from build123d import *

# Parameters (mm, degrees)
SKETCH1_R           = 2.286
BOSS_EXTRUDE1_DEPTH = 6.35
CHAMFER1_SIZE       = 17.78
CHAMFER1_SIZE2      = 26.652616032
FILLET1_R           = 3.81


with BuildPart() as part:
    # Sketch1 → Boss-Extrude1 (new body)
    with BuildSketch(Plane.XY):
        Polygon((-34.167492812, 55.206788795), (-6.35, 37.482986116), (-6.35, -6.35), (6.35, -6.35), (6.35, 44.45), (-27.343211205, 65.917492812), align=None)
        Circle(SKETCH1_R, mode=Mode.SUBTRACT)
        with Locations((0, 38.1)):
            Circle(SKETCH1_R, mode=Mode.SUBTRACT)
        with Locations((-25.4, 57.15)):
            Circle(SKETCH1_R, mode=Mode.SUBTRACT)
    extrude(amount=BOSS_EXTRUDE1_DEPTH)

    # Chamfer1
    chamfer1_edges = [part.edges().sort_by_distance(p)[0] for p in [
        (-6.35, 37.482986116, 3.175),
    ]]
    chamfer1_side = [part.faces().sort_by_distance(p)[0] for p in [
        (-20.258746406, 46.344887456, 3.175),
    ]]
    chamfer(chamfer1_edges, length=CHAMFER1_SIZE, length2=CHAMFER1_SIZE2, reference=chamfer1_side[0])

    # Fillet1
    fillet1_edges = [part.edges().sort_by_distance(p)[0] for p in [
        (-27.343211205, 65.917492812, 3.175),
        (6.35, 44.45, 3.175),
        (6.35, -6.35, 3.175),
        (-6.35, -6.35, 3.175),
        (-34.167492812, 55.206788795, 3.175),
        (-6.35, 10.830370085, 3.175),
        (-21.344985624, 47.036980366, 3.175),
    ]]
    fillet(fillet1_edges, radius=FILLET1_R)


solid = part.part
Check sheet for the modelled part. Datum: model origin and axes. Units: mm. A direction names the side the tool comes from. Give positions to 0.01 mm unless a question says otherwise; leave off trailing zeros. Loops run counter-clockwise (first coordinate to the right, second up) from the corner with the lowest first, then second, coordinate; pieces in that order, holes last. Notation, with made-up numbers: M -25,21 L 7,21 A26 cw 7,35 Z; hole C 69,-0.75 d9. An arc over 180 degrees is marked long. Answer as a JSON object with one key per item and string values. Group by question number.
Q1. Cross-section at A-A on y = 0. Record the cut outline in (x, z).
Q2. Go/stop test with flat-tipped pins: P1, Ø5.5, axis at x = 0, y = 38.1, coming from the -Z side; P2, Ø2, axis at y = 10, z = 5, coming from the -X side. Record where each tip stops, or that it passes through.
Q3. Material ranges on line 1 along Y through (x, z) = (-2, 2.75); line 2 along Y through (x, z) = (0, 3.5); line 3 along X through (y, z) = (39, 4.25), recorded low to high. Write a range as [from, to].
Q4. Cross-section at D-D on y = 52. Record the cut outline in (x, z).
Q5. Access from +Z, -Z, +X, -X, +Y, -Y to the whole of each face (thin tool, end or side, straight path). Record for faces 1 (the cylindrical face through (5.204, -5.264, 3.219)), 2 (the flat face through (-6.35, 4, 3)).
Q6. Release check for a two-part mould opening along X. For faces 3 (the flat face through (-9, 30, 0)), 4 (the cylindrical face through (-6.425, 10.826, 3.219)), 5 (the cylindrical face through (-23.22, 57.84, 3.13)) record: released by +X, released by -X, zero draft, split by the parting line, or undercut.
Q7. Cross-section at C-C on x = -25.4. Record the cut outline in (y, z), then the cut area to 3 significant figures.
Q8. Cross-section at B-B on z = 2. Record the cut outline in (x, y).
Evaluation:
{
 "1": {"outline": "M -6.35,0 L -2.29,0 L -2.29,6.35 L -6.35,6.35 Z; M 2.29,0 L 6.35,0 L 6.35,6.35 L 2.29,6.35 Z"},
 "2": {"P1": "stops at z = 0", "P2": "stops at x = -6.46"},
 "3": {"line 1": "y = [-6.35, -1.11], [1.11, 36.99], [39.21, 49.77]", "line 2": "y = [-6.35, -2.29], [2.29, 35.81], [40.39, 48.5]", "line 3": "x = [-18.02, -2.1], [2.1, 6.35]"},
 "4": {"outline": "M -29.13,0 L -5.5,0 L -5.5,6.35 L -29.13,6.35 Z"},
 "5": {"face 1": "+Z, -Z, +X, -Y", "face 2": "+Z, -Z, -X, -Y"},
 "6": {"face 3": "zero draft", "face 4": "released by -X", "face 5": "undercut"},
 "7": {"outline": "M 49.62,0 L 54.86,0 L 54.86,6.35 L 49.62,6.35 Z; M 59.44,0 L 64.39,0 L 64.39,6.35 L 59.44,6.35 Z", "area": "64.7 mm2"},
 "8": {"outline": "M -32.12,58.42 A3.81 ccw -30.95,53.16 L -22.36,47.68 A3.81 cw -20.89,45.93 L -6.64,11.53 A3.81 cw -6.35,10.07 L -6.35,-2.54 A3.81 ccw -2.54,-6.35 L 2.54,-6.35 A3.81 ccw 6.35,-2.54 L 6.35,42.36 A3.81 ccw 4.59,45.57 L -24.13,63.87 A3.81 ccw -29.39,62.7 Z; hole C -25.4,57.15 d4.57; hole C 0,0 d4.57; hole C 0,38.1 d4.57"}
}
